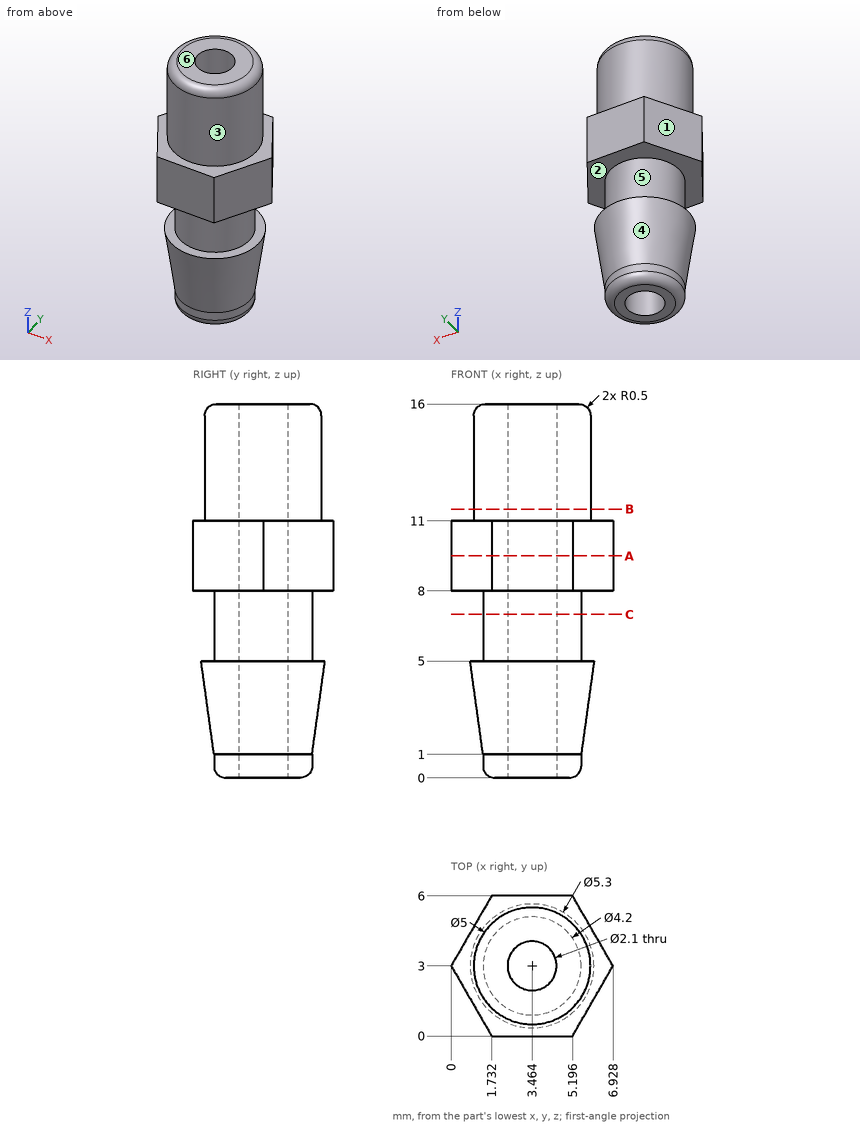
For this review, use the dimensioned drawing (mm, ordinates from the lowest corner) and the shaded views. A direction names the side the tool comes from. Give positions to 0.01 mm unless a question says otherwise; leave off trailing zeros. Order: outer loops, then holes, each group sorted by start corner. A loop starts at its lowest first (then second) coordinate and runs counter-clockwise, first axis right, second up.
1) Take a section at A-A (z = 9.5). Give the boundary of the cut face in (x, y).
2) Take a section at B-B (z = 11.5). Give the boundary of the cut face in (x, y).
3) Take a section at C-C (z = 7). Give the boundary of the cut face in (x, y).
4) For the marked faces 1 and 2, list the 3-axis set-ups (+Z, -Z, +X, -X, +Y, -Y) from which the entire face can be reached by the end or side of a thin tool; tool diameter is ignored.
5) Wall thickness on line 1 (Z direction, x = 2.75, y = 1.5); line 2 (Z direction, x = 0.5, y = 2.35); line 3 (Y direction, x = 3.5, z = 3.25): over which ranges is each line inside the solid? List them lowest first.
6) The part is to be moulded in two halves that separate along Z. For the marked faces 3, 4, 5 and 6, say which applies: released by +Z, released by -Z, zero draft, split by the parting line, or undercut.
7) Insertion check: pin 1 (1.5 mm diameter, centred on y = 4.5, z = 3, fed in from -X); pin 2 (1 mm diameter, centred on y = 5, z = 4, fed in from -X); pin 3 (3 mm diameter, centred on x = 2.5, y = 4.5, fed in from -Z); pin 4 (1.5 mm diameter, centred on y = 1.5, z = 10, fed in from -X). Each pin has a flat end and moves straight along its axis. Give the tip position at first contact, or say it passes through.
Derived:
1. outline: (0, 3) - (1.73, 0) - (5.2, 0) - (6.93, 3) - (5.2, 6) - (1.73, 6) - close; hole circle Ø2.1 at (3.46, 3)
2. outline: circle Ø5 at (3.46, 3); hole circle Ø2.1 at (3.46, 3)
3. outline: circle Ø4.2 at (3.46, 3); hole circle Ø2.1 at (3.46, 3)
4. face 1: +Z, -Z, -X, +Y
4. face 2: none
5. line 1: z = 0 to 16
5. line 2: z = 8 to 11
5. line 3: y = 0.59 to 1.95, 4.05 to 5.41
6. face 3: zero draft
6. face 4: released by -Z
6. face 5: undercut
6. face 6: released by +Z
7. pin 1: stops at x = 1.19
7. pin 2: stops at x = 1.44
7. pin 3: stops at z = 0
7. pin 4: stops at x = 0.43
